Geometry check sheet. Reference: the model listing, model coordinates, mm. Coordinates: 2 decimals unless noted, no trailing zeros. Write each loop counter-clockwise with the first axis right and the second up, starting at its lowest first coordinate (ties: lowest second). Pieces come first, ordered by that corner, then holes. Notation, with made-up numbers: M -21.5,70.5 L -13.5,70.5 A7 cw -13.5,78.5 Z; hole C 70.5,57 d10. An arc over 180 degrees is marked long. Answer as a JSON object with one key per item and string values. Group by question number.
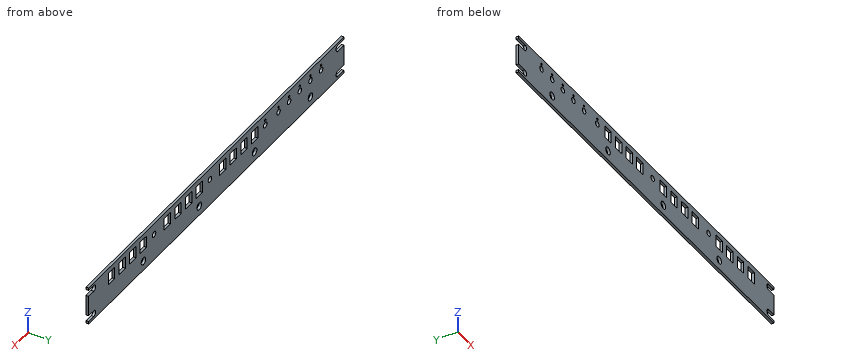
```python
from build123d import *

# Parameters (mm, degrees)
F0_R     = 4.25
F0_W     = 12
F0_H     = 14
F0_R_2   = 3.25
F1_DEPTH = 3


with BuildPart() as f1:
    # F0 (on Front) → F1 (new body)
    with BuildSketch(Plane.XZ):
        with BuildLine():
            Line((235.9719324717, -52.8782820007), (-244.0280675283, -52.8782820007))
            Line((-244.0280675283, -52.8782820007), (-244.0280675283, -55.8782820007))
            Line((-244.0280675283, -55.8782820007), (-230.8552050385, -55.8782820007))
            ThreePointArc((-230.8552050385, -55.8782820007), (-229.0280675283, -58.9526162523), (-230.8552050385, -62.0269505038))
            Line((-230.8552050385, -62.0269505038), (-230.8552050385, -63.012175262))
            Line((-230.8552050385, -63.012175262), (-244.0280675283, -63.012175262))
            Line((-244.0280675283, -63.012175262), (-244.0280675283, -86.8791321319))
            Line((-244.0280675283, -86.8791321319), (-232.6052050385, -86.8791321319))
            ThreePointArc((-232.6052050385, -86.8791321319), (-229.0280675283, -90.3782820007), (-232.6052050385, -93.8774318695))
            Line((-232.6052050385, -93.8774318695), (-232.6052050385, -93.8782820007))
            Line((-232.6052050385, -93.8782820007), (-244.0280675283, -93.8782820007))
            Line((-244.0280675283, -93.8782820007), (-244.0280675283, -96.8782820007))
            Line((-244.0280675283, -96.8782820007), (235.9719324717, -96.8782820007))
            Line((235.9719324717, -96.8782820007), (235.9719324717, -93.8782820007))
            Line((235.9719324717, -93.8782820007), (226.299069982, -93.8782820007))
            Line((226.299069982, -93.8782820007), (226.299069982, -93.8774318695))
            ThreePointArc((226.299069982, -93.8774318695), (222.7219324717, -90.3782820007), (226.299069982, -86.8791321319))
            Line((226.299069982, -86.8791321319), (235.9719324717, -86.8791321319))
            Line((235.9719324717, -86.8791321319), (235.9719324717, -63.012175262))
            Line((235.9719324717, -63.012175262), (226.299069982, -63.012175262))
            Line((226.299069982, -63.012175262), (226.299069982, -62.8765817383))
            ThreePointArc((226.299069982, -62.8765817383), (222.7219324717, -59.3774318695), (226.299069982, -55.8782820007))
            Line((226.299069982, -55.8782820007), (235.9719324717, -55.8782820007))
            Line((235.9719324717, -55.8782820007), (235.9719324717, -52.8782820007))
        make_face()
        with Locations((-76.0280675283, -85.8782820007)):
            Circle(F0_R, mode=Mode.SUBTRACT)
        with Locations((-181.0280675283, -85.8782820007)):
            Circle(F0_R, mode=Mode.SUBTRACT)
        with Locations((27.9719324717, -85.8782820007)):
            Circle(F0_R, mode=Mode.SUBTRACT)
        with Locations((132.9719324717, -85.8782820007)):
            Circle(F0_R, mode=Mode.SUBTRACT)
        with BuildLine():
            Line((-207.0280675283, -72.8782820007), (-207.0280675283, -58.8782820007))
            Line((-207.0280675283, -58.8782820007), (-201.7780675283, -58.8782820007))
            ThreePointArc((-201.7780675283, -58.8782820007), (-201.0280675283, -58.6282820007), (-200.2780675283, -58.8782820007))
            Line((-200.2780675283, -58.8782820007), (-195.0280675283, -58.8782820007))
            Line((-195.0280675283, -58.8782820007), (-195.0280675283, -72.8782820007))
            Line((-195.0280675283, -72.8782820007), (-207.0280675283, -72.8782820007))
        make_face(mode=Mode.SUBTRACT)
        with BuildLine():
            Line((-187.0280675283, -72.8782820007), (-187.0280675283, -58.8782820007))
            Line((-187.0280675283, -58.8782820007), (-181.7780675283, -58.8782820007))
            ThreePointArc((-181.7780675283, -58.8782820007), (-181.0280675283, -58.6282820007), (-180.2780675283, -58.8782820007))
            Line((-180.2780675283, -58.8782820007), (-175.0280675283, -58.8782820007))
            Line((-175.0280675283, -58.8782820007), (-175.0280675283, -72.8782820007))
            Line((-175.0280675283, -72.8782820007), (-187.0280675283, -72.8782820007))
        make_face(mode=Mode.SUBTRACT)
        with BuildLine():
            Line((-167.0280675283, -72.8782820007), (-167.0280675283, -58.8782820007))
            Line((-167.0280675283, -58.8782820007), (-161.7780675283, -58.8782820007))
            ThreePointArc((-161.7780675283, -58.8782820007), (-161.0280675283, -58.6282820007), (-160.2780675283, -58.8782820007))
            Line((-160.2780675283, -58.8782820007), (-155.0280675283, -58.8782820007))
            Line((-155.0280675283, -58.8782820007), (-155.0280675283, -72.8782820007))
            Line((-155.0280675283, -72.8782820007), (-167.0280675283, -72.8782820007))
        make_face(mode=Mode.SUBTRACT)
        with BuildLine():
            Line((-147.0280675283, -72.8782820007), (-147.0280675283, -58.8782820007))
            Line((-147.0280675283, -58.8782820007), (-141.7780675283, -58.8782820007))
            ThreePointArc((-141.7780675283, -58.8782820007), (-141.0280675283, -58.6282820007), (-140.2780675283, -58.8782820007))
            Line((-140.2780675283, -58.8782820007), (-135.0280675283, -58.8782820007))
            Line((-135.0280675283, -58.8782820007), (-135.0280675283, -72.8782820007))
            Line((-135.0280675283, -72.8782820007), (-147.0280675283, -72.8782820007))
        make_face(mode=Mode.SUBTRACT)
        with BuildLine():
            Line((-127.0280675283, -72.8782820007), (-127.0280675283, -58.8782820007))
            Line((-127.0280675283, -58.8782820007), (-121.7780675283, -58.8782820007))
            ThreePointArc((-121.7780675283, -58.8782820007), (-121.0280675283, -58.6282820007), (-120.2780675283, -58.8782820007))
            Line((-120.2780675283, -58.8782820007), (-115.0280675283, -58.8782820007))
            Line((-115.0280675283, -58.8782820007), (-115.0280675283, -72.8782820007))
            Line((-115.0280675283, -72.8782820007), (-127.0280675283, -72.8782820007))
        make_face(mode=Mode.SUBTRACT)
        with BuildLine():
            Line((-102.0280675283, -72.8782820007), (-102.0280675283, -58.8782820007))
            Line((-102.0280675283, -58.8782820007), (-96.7780675283, -58.8782820007))
            ThreePointArc((-96.7780675283, -58.8782820007), (-96.0280675283, -58.6282820007), (-95.2780675283, -58.8782820007))
            Line((-95.2780675283, -58.8782820007), (-90.0280675283, -58.8782820007))
            Line((-90.0280675283, -58.8782820007), (-90.0280675283, -72.8782820007))
            Line((-90.0280675283, -72.8782820007), (-102.0280675283, -72.8782820007))
        make_face(mode=Mode.SUBTRACT)
        with Locations((-76.0280675283, -65.8782820007)):
            Rectangle(F0_W, F0_H, mode=Mode.SUBTRACT)
        with Locations((-56.0280675283, -65.8782820007)):
            Rectangle(F0_W, F0_H, mode=Mode.SUBTRACT)
        with Locations((-36.0280675283, -65.8782820007)):
            Rectangle(F0_W, F0_H, mode=Mode.SUBTRACT)
        with Locations((-16.0280675283, -65.8782820007)):
            Rectangle(F0_W, F0_H, mode=Mode.SUBTRACT)
        with Locations((7.9719324717, -65.8782820007)):
            Rectangle(F0_W, F0_H, mode=Mode.SUBTRACT)
        with Locations((27.9719324717, -65.8782820007)):
            Rectangle(F0_W, F0_H, mode=Mode.SUBTRACT)
        with Locations((47.9719324717, -65.8782820007)):
            Rectangle(F0_W, F0_H, mode=Mode.SUBTRACT)
        with Locations((67.9719324717, -65.8782820007)):
            Rectangle(F0_W, F0_H, mode=Mode.SUBTRACT)
        with Locations((87.9719324717, -65.8782820007)):
            Rectangle(F0_W, F0_H, mode=Mode.SUBTRACT)
        with Locations((112.9719324717, -65.8782820007)):
            Rectangle(F0_W, F0_H, mode=Mode.SUBTRACT)
        with Locations((132.9719324717, -65.8782820007)):
            Rectangle(F0_W, F0_H, mode=Mode.SUBTRACT)
        with Locations((152.9719324717, -65.8782820007)):
            Rectangle(F0_W, F0_H, mode=Mode.SUBTRACT)
        with Locations((172.9719324717, -65.8782820007)):
            Rectangle(F0_W, F0_H, mode=Mode.SUBTRACT)
        with Locations((192.9719324717, -65.8782820007)):
            Rectangle(F0_W, F0_H, mode=Mode.SUBTRACT)
        with BuildLine():
            Line((-201.7780675283, -58.8782820007), (-207.0280675283, -58.8782820007))
            Line((-207.0280675283, -58.8782820007), (-207.0280675283, -72.8782820007))
            Line((-207.0280675283, -72.8782820007), (-195.0280675283, -72.8782820007))
            Line((-195.0280675283, -72.8782820007), (-195.0280675283, -58.8782820007))
            Line((-195.0280675283, -58.8782820007), (-200.2780675283, -58.8782820007))
            ThreePointArc((-200.2780675283, -58.8782820007), (-199.9100335395, -59.3192650063), (-199.7780675283, -59.8782820007))
            ThreePointArc((-199.7780675283, -59.8782820007), (-201.5870845227, -60.9963159894), (-201.7780675283, -58.8782820007))
        make_face()
        with Locations((-201.0280675283, -65.8782820007)):
            Circle(F0_R_2, mode=Mode.SUBTRACT)
        with BuildLine():
            Line((-181.7780675283, -58.8782820007), (-187.0280675283, -58.8782820007))
            Line((-187.0280675283, -58.8782820007), (-187.0280675283, -72.8782820007))
            Line((-187.0280675283, -72.8782820007), (-175.0280675283, -72.8782820007))
            Line((-175.0280675283, -72.8782820007), (-175.0280675283, -58.8782820007))
            Line((-175.0280675283, -58.8782820007), (-180.2780675283, -58.8782820007))
            ThreePointArc((-180.2780675283, -58.8782820007), (-179.9100335395, -59.3192650063), (-179.7780675283, -59.8782820007))
            ThreePointArc((-179.7780675283, -59.8782820007), (-181.5870845227, -60.9963159894), (-181.7780675283, -58.8782820007))
        make_face()
        with Locations((-181.0280675283, -65.8782820007)):
            Circle(F0_R_2, mode=Mode.SUBTRACT)
        with BuildLine():
            Line((-121.7780675283, -58.8782820007), (-127.0280675283, -58.8782820007))
            Line((-127.0280675283, -58.8782820007), (-127.0280675283, -72.8782820007))
            Line((-127.0280675283, -72.8782820007), (-115.0280675283, -72.8782820007))
            Line((-115.0280675283, -72.8782820007), (-115.0280675283, -58.8782820007))
            Line((-115.0280675283, -58.8782820007), (-120.2780675283, -58.8782820007))
            ThreePointArc((-120.2780675283, -58.8782820007), (-119.9100335395, -59.3192650063), (-119.7780675283, -59.8782820007))
            ThreePointArc((-119.7780675283, -59.8782820007), (-121.5870845227, -60.9963159894), (-121.7780675283, -58.8782820007))
        make_face()
        with Locations((-121.0280675283, -65.8782820007)):
            Circle(F0_R_2, mode=Mode.SUBTRACT)
        with BuildLine():
            Line((-96.7780675283, -58.8782820007), (-102.0280675283, -58.8782820007))
            Line((-102.0280675283, -58.8782820007), (-102.0280675283, -72.8782820007))
            Line((-102.0280675283, -72.8782820007), (-90.0280675283, -72.8782820007))
            Line((-90.0280675283, -72.8782820007), (-90.0280675283, -58.8782820007))
            Line((-90.0280675283, -58.8782820007), (-95.2780675283, -58.8782820007))
            ThreePointArc((-95.2780675283, -58.8782820007), (-94.9100335395, -59.3192650063), (-94.7780675283, -59.8782820007))
            ThreePointArc((-94.7780675283, -59.8782820007), (-96.5870845227, -60.9963159894), (-96.7780675283, -58.8782820007))
        make_face()
        with Locations((-96.0280675283, -65.8782820007)):
            Circle(F0_R_2, mode=Mode.SUBTRACT)
        with Locations((7.9719324717, -65.8782820007)):
            Rectangle(F0_W, F0_H)
        with Locations((7.9719324717, -65.8782820007)):
            Circle(F0_R_2, mode=Mode.SUBTRACT)
        with Locations((112.9719324717, -65.8782820007)):
            Rectangle(F0_W, F0_H)
        with Locations((112.9719324717, -65.8782820007)):
            Circle(F0_R_2, mode=Mode.SUBTRACT)
        with BuildLine():
            Line((-161.7780675283, -58.8782820007), (-167.0280675283, -58.8782820007))
            Line((-167.0280675283, -58.8782820007), (-167.0280675283, -72.8782820007))
            Line((-167.0280675283, -72.8782820007), (-155.0280675283, -72.8782820007))
            Line((-155.0280675283, -72.8782820007), (-155.0280675283, -58.8782820007))
            Line((-155.0280675283, -58.8782820007), (-160.2780675283, -58.8782820007))
            ThreePointArc((-160.2780675283, -58.8782820007), (-159.9100335395, -59.3192650063), (-159.7780675283, -59.8782820007))
            ThreePointArc((-159.7780675283, -59.8782820007), (-161.5870845227, -60.9963159894), (-161.7780675283, -58.8782820007))
        make_face()
        with Locations((-161.0280675283, -65.8782820007)):
            Circle(F0_R_2, mode=Mode.SUBTRACT)
        with BuildLine():
            Line((-141.7780675283, -58.8782820007), (-147.0280675283, -58.8782820007))
            Line((-147.0280675283, -58.8782820007), (-147.0280675283, -72.8782820007))
            Line((-147.0280675283, -72.8782820007), (-135.0280675283, -72.8782820007))
            Line((-135.0280675283, -72.8782820007), (-135.0280675283, -58.8782820007))
            Line((-135.0280675283, -58.8782820007), (-140.2780675283, -58.8782820007))
            ThreePointArc((-140.2780675283, -58.8782820007), (-139.9100335395, -59.3192650063), (-139.7780675283, -59.8782820007))
            ThreePointArc((-139.7780675283, -59.8782820007), (-141.5870845227, -60.9963159894), (-141.7780675283, -58.8782820007))
        make_face()
        with Locations((-141.0280675283, -65.8782820007)):
            Circle(F0_R_2, mode=Mode.SUBTRACT)
    extrude(amount=F1_DEPTH)


solid = f1.part
```
1) Section check A-A (x = 90). Record the cut outline in (y, z).
2) Material ranges on probe 1 along Z at (x, y) = (83.5, -2.2); probe 2 along Z at (x, y) = (-74, -1.5); probe 3 along X at (y, z) = (-1.65, -88), recorded low to high. Write a range as [from, to].
3) Section check B-B (y = -1.65). State how many separate pieces and enclosed holes the cut face has, then the cut area to 3 significant figures.
Entries:
{
 "1": {"outline": "M -3,-96.88 L 0,-96.88 L 0,-72.88 L -3,-72.88 Z; M -3,-58.88 L 0,-58.88 L 0,-52.88 L -3,-52.88 Z"},
 "2": {"probe 1": "[-96.88, -72.88], [-58.88, -52.88]", "probe 2": "[-96.88, -89.61], [-82.14, -72.88], [-58.88, -52.88]", "probe 3": "[-229.96, -184.71], [-177.35, -79.71], [-72.35, 24.29], [31.65, 129.29], [136.65, 223.65]"},
 "3": {"separate pieces": "1", "enclosed holes": "30", "area": "18,200 mm^2"}
}
